Source: CAD feature listing. Evaluate the final solid. Frame: model axes, mm. Face numbers are marked on the shaded views. A direction names the side the tool comes from. Round coordinates to 2 decimals unless told otherwise and drop trailing zeros. Write each loop counter-clockwise with the first axis right and the second up, starting at its lowest first coordinate (ties: lowest second). Pieces come first, ordered by that corner, then holes. Notation, with made-up numbers: M 54,50 L 100,50 A24 cw 100,74 Z; hole C 83,26.25 d1. An arc over 180 degrees is marked long. Answer in a Markdown table with one row per item. Add a question column.
Item 1: Set-up query: the marked faces 4 and 5. Return all of +Z, -Z, +X, -X, +Y, -Y with unobstructed straight access to the full face (end or side cutting, diameter ignored); none if empty.
Item 2: Cut plane A-A on x = 21. Return loops of the section in (y, z), and give its area (3 significant figures).
Item 3: Material intervals for probe 1 along Y at (x, z) = (21.5, 48); probe 2 along Y at (x, z) = (53, 1.25); probe 3 along X at (y, z) = (46, 47.5), sorted ascending.
Item 4: Contact query for flat-ended pins moving along their axis: pin 1 (2 mm diameter, centred on x = 40.5, z = 35.5, fed in from -Y); pin 2 (6 mm diameter, centred on x = 28, y = 20.5, fed in from +Z); pin 3 (5 mm diameter, centred on x = 5.54, y = 18.24, fed in from +Z). Output: stop coordinate, or through.
Item 5: Cut plane C-C on x = 10. Return loops of the section in (y, z), and give its area (3 significant figures).
Item 6: Cut plane B-B on z = 26.5. Return loops of the section in (x, y), and give its area (3 significant figures).
Item 7: Mould query, pull axis Y, two halves, no side actions, for the marked faces 1, 2 and 3. Classes: released by +Y, released by -Y, zero draft, split by the parting line, or undercut.
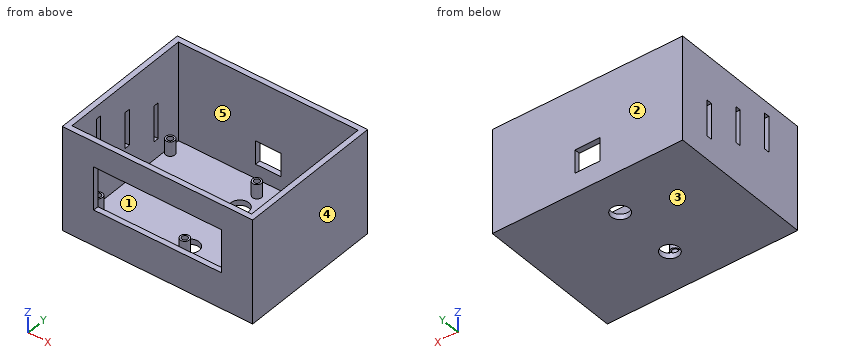
Autodesk Inventor part; units mm, degrees
ref_plane "YZ Plane" through (0, 0, 0) normal (1, 0, 0) x (0, 1, 0)
ref_plane "XZ Plane" through (0, 0, 0) normal (0, 1, 0) x (-1, 0, 0)
ref_plane "XY Plane" through (0, 0, 0) normal (0, 0, 1) x (1, 0, 0)
sketch "Sketch1" plane through (0, 0, 0) normal (0, 0, 1) x (1, 0, 0)
  line L0 (0, 0) -> (106, 0)
  line L1 (106, 0) -> (106, 81)
  line L2 (106, 81) -> (0, 81)
  line L3 (0, 81) -> (0, 0)
  dimension "d0" = 106
  dimension "d1" = 81
extrude "Extrusion1" add sketch "Sketch1" along normal blind 58
shell "Shell1" thickness 3 removed faces 1 at (70.6667, 27, 58)
sketch "Sketch2" plane through (0, 0, 0) normal (0, -1, 0) x (1, 0, 0)
  line L0 (17.5, 20) -> (88.5, 20)
  line L1 (88.5, 20) -> (88.5, 44)
  line L2 (88.5, 44) -> (17.5, 44)
  line L3 (17.5, 44) -> (17.5, 20)
  line L4 (0, 0) -> (0, 58)
  line L5 (0, 0) -> (106, 0)
  dimension "d5" = 71
  dimension "d6" = 24
  dimension "d7" = 17.5
  dimension "d8" = 20
extrude "Extrusion2" cut sketch "Sketch2" against normal blind 3
sketch "Sketch3" plane through (0, 81, 0) normal (0, 1, 0) x (1, 0, 0)
  line L0 (60, -24) -> (46, -24)
  line L1 (46, -24) -> (46, -11)
  line L2 (46, -11) -> (60, -11)
  line L3 (60, -11) -> (60, -24)
  line L4 (106, 0) -> (106, -58)
  line L5 (106, 0) -> (0, 0)
  dimension "d11" = 14
  dimension "d12" = 13
  dimension "d13" = 46
  dimension "d14" = 11
extrude "Extrusion3" cut sketch "Sketch3" against normal blind 3
sketch "Sketch4" plane through (0, 0, 0) normal (-1, 0, 0) x (0, 0, 1)
  line L0 (33, 63.75) -> (13, 63.75)
  line L1 (13, 63.75) -> (13, 60.75)
  line L2 (13, 60.75) -> (33, 60.75)
  line L3 (33, 60.75) -> (33, 63.75)
  line L4 (42, 43.5) -> (22, 43.5)
  line L5 (22, 43.5) -> (22, 40.5)
  line L6 (22, 40.5) -> (42, 40.5)
  line L7 (42, 40.5) -> (42, 43.5)
  line L8 (31, 23.25) -> (51, 23.25)
  line L9 (51, 23.25) -> (51, 20.25)
  line L10 (51, 20.25) -> (31, 20.25)
  line L11 (31, 20.25) -> (31, 23.25)
  line L12 (0, 81) -> (0, 0)
  line L13 (0, 81) -> (58, 81)
  line L14 (0, 0) -> (58, 0)
  dimension "d17" = 20
  dimension "d18" = 3
  dimension "d19" = 20
  dimension "d20" = 3
  dimension "d21" = 20
  dimension "d22" = 3
  dimension "d23" = 13
  dimension "d24" = 22
  dimension "d25" = 31
  dimension "d90" = 20.25
  dimension "d91" = 40.5
  dimension "d92" = 60.75
sketch "Sketch5" plane through (3, 78, 3) normal (0, 0, 1) x (1, 0, 0)
  circle A0 centre (2.54, -59.76) radius 2.5
  line L0 (0, 0) -> (0, -75)
  line L1 (0, -75) -> (100, -75)
  circle A1 centre (2.54, -8.96) radius 2.5
  circle A2 centre (50.8, -8.96) radius 2.5
  circle A3 centre (50.8, -59.76) radius 2.5
  point P0 (-3, -78)
  dimension "d28" = 5
  dimension "d29" = 2.54
  dimension "d30" = 15.24
  dimension "d31" = 5
  dimension "d32" = 2.54
  dimension "d33" = 66.04
  dimension "d34" = 5
  dimension "d35" = 50.8
  dimension "d36" = 66.04
  dimension "d37" = 5
  dimension "d38" = 50.8
  dimension "d39" = 15.24
extrude "Extrusion4" add sketch "Sketch5" along normal blind 8
sketch "Sketch6" plane through (5.54, 69.04, 11) normal (0, 0, 1) x (1, 0, 0)
  point P0 (-5.54, -69.04)
  point P1 (0, 0)
sketch "Sketch7" plane through (5.54, 18.24, 11) normal (0, 0, 1) x (1, 0, 0)
  circle A0 centre (48.26, 0) radius 2.5
  point P0 (-5.54, -18.24)
  point P1 (0, 0)
sketch "Sketch8" plane through (53.8, 69.04, 11) normal (0, 0, 1) x (1, 0, 0)
  point P0 (-53.8, -69.04)
  point P1 (0, 0)
hole "Hole1" at (5.54, 69.04, 11) direction (0, 0, -1) diameter 3.2 depth 8
hole "Hole2" at (53.8, 69.04, 11) direction (0, 0, -1) diameter 3.2 depth 8
hole "Hole3" at (5.54, 18.24, 11) direction (0, 0, -1) diameter 3.2 depth 8
sketch "Sketch9" plane through (53.8, 18.24, 11) normal (0, 0, 1) x (1, 0, 0)
  point P0 (-53.8, -18.24)
  point P1 (0, 0)
hole "Hole4" at (53.8, 18.24, 11) direction (0, 0, -1) diameter 3.2 depth 8
sketch "Sketch10" plane through (3, 3, 3) normal (0, 1, 0) x (1, 0, 0)
  line L0 (85.5, -5) -> (95.5, -5)
  line L1 (95.5, -5) -> (95.5, 0)
  line L2 (95.5, 0) -> (85.5, 0)
  line L3 (85.5, 0) -> (85.5, -5)
  line L4 (85.5, -17) -> (85.5, -41)
  line L5 (0, 0) -> (100, 0)
  line L6 (14.5, -5) -> (4.5, -5)
  line L7 (4.5, -5) -> (4.5, 0)
  line L8 (4.5, 0) -> (14.5, 0)
  line L9 (14.5, 0) -> (14.5, -5)
  line L10 (14.5, -41) -> (14.5, -17)
  point P0 (-3, 3)
  dimension "d70" = 10
  dimension "d71" = 5
  dimension "d72" = 0
  dimension "d74" = 10
  dimension "d75" = 5
  dimension "d76" = 0
  dimension "d77" = 0
  dimension "d80" = 0
extrude "Extrusion5" add sketch "Sketch10" along normal blind 3
sketch "Sketch11" plane through (0, 0, 0) normal (0, 0, -1) x (-1, 0, 0)
  circle A0 centre (-53, 58) radius 5
  circle A1 centre (-53, 23) radius 5
  line L0 (-106, 0) -> (-106, 81)
  line L1 (-106, 81) -> (0, 81)
  line L2 (0, 0) -> (-106, 0)
  dimension "d81" = 10
  dimension "d82" = 10
  dimension "d83" = 53
  dimension "d84" = 53
  dimension "d85" = 23
  dimension "d86" = 23
extrude "Extrusion6" cut sketch "Sketch11" against normal blind 3.5
extrude "Extrusion7" cut sketch "Sketch4" against normal blind 3.5
properties part number "air-monitor_enclosure"
Results below:
| question | item | result |
|---|---|---|
| 1 | face 4 | +Z, -Z, +X, +Y, -Y |
| 1 | face 5 | +Z |
| 2 | outline | M 0,0 L 81,0 L 81,58 L 78,58 L 78,3 L 3,3 L 3,20 L 0,20 Z; M 0,44 L 3,44 L 3,58 L 0,58 Z |
| 2 | area | 501 mm2 |
| 3 | probe 1 | 0 to 3, 78 to 81 |
| 3 | probe 2 | 0 to 18, 28 to 53, 63 to 81 |
| 3 | probe 3 | 0 to 3, 103 to 106 |
| 4 | pin 1 | y = 78 |
| 4 | pin 2 | z = 3 |
| 4 | pin 3 | z = 11 |
| 5 | outline | M 0,0 L 81,0 L 81,58 L 78,58 L 78,3 L 6,3 L 6,8 L 3,8 L 3,58 L 0,58 Z |
| 5 | area | 588 mm2 |
| 6 | outline | M 0,0 L 17.5,0 L 17.5,3 L 3,3 L 3,40.5 L 0,40.5 Z; M 0,43.5 L 3,43.5 L 3,60.75 L 0,60.75 Z; M 0,63.75 L 3,63.75 L 3,78 L 103,78 L 103,3 L 88.5,3 L 88.5,0 L 106,0 L 106,81 L 0,81 Z |
| 6 | area | 855 mm2 |
| 7 | face 1 | undercut |
| 7 | face 2 | released by +Y |
| 7 | face 3 | zero draft |
